Here's how the part is built. I have some questions about the finished solid (model axes, mm). A direction names the side the tool comes from. Round coordinates to 2 decimals unless told otherwise and drop trailing zeros. Loops run counter-clockwise (first coordinate to the right, second up) from the corner with the lowest first, then second, coordinate; pieces in that order, holes last. Notation, with made-up numbers: M 44,-0.5 L 90,-0.5 A22 cw 90,36.5 Z; hole C -33,54.25 d7. An arc over 180 degrees is marked long. One line per question, with ' | ' between items. Start each with the question number.
```python
from build123d import *

# Parameters (mm, degrees)
F0_W     = 76.2
F0_H     = 44.45
F1_DEPTH = 25.4
F2_W     = 25.4
F2_H     = 31.75
F3_DEPTH = 25.4
F5_DEPTH = 25.4
F7_DEPTH = 25.4
F9_DEPTH = 25.4


with BuildPart() as f1:
    # F0 (on Front) → F1 (new body)
    with BuildSketch(Plane.XZ):
        with Locations((38.1, 22.225)):
            Rectangle(F0_W, F0_H)
    extrude(amount=F1_DEPTH)

    # F2 (on face) → F3 (cut)
    with BuildSketch(Plane.XZ.offset(25.4)):
        with Locations((12.7, 28.575)):
            Rectangle(F2_W, F2_H)
        with Locations((63.5, 28.575)):
            Rectangle(F2_W, F2_H)
    extrude(amount=-F3_DEPTH, mode=Mode.SUBTRACT)

    # F4 (on face) → F5 (cut)
    with BuildSketch(Plane.YZ.offset(50.8)):
        with BuildLine():
            Line((-12.7, 28.575), (-12.7, 34.925))
            ThreePointArc((-12.7, 34.925), (-17.1901280605, 33.0651280605), (-19.05, 28.575))
            Line((-19.05, 28.575), (-12.7, 28.575))
        make_face()
        with BuildLine():
            ThreePointArc((-6.35, 28.575), (-8.2098719395, 33.0651280605), (-12.7, 34.925))
            Line((-12.7, 34.925), (-12.7, 28.575))
            Line((-12.7, 28.575), (-6.35, 28.575))
        make_face()
        with BuildLine():
            Line((-6.35, 28.575), (-12.7, 28.575))
            Line((-12.7, 28.575), (-12.7, 22.225))
            ThreePointArc((-12.7, 22.225), (-8.2098719395, 24.0848719395), (-6.35, 28.575))
        make_face()
        with BuildLine():
            Line((-12.7, 22.225), (-12.7, 28.575))
            Line((-12.7, 28.575), (-19.05, 28.575))
            ThreePointArc((-19.05, 28.575), (-17.1901280605, 24.0848719395), (-12.7, 22.225))
        make_face()
        with BuildLine():
            Line((-12.7, 44.3012688375), (-12.7, 44.45))
            Line((-12.7, 44.45), (-25.4, 44.45))
            Line((-25.4, 44.45), (-25.4, 37.8499949622))
            ThreePointArc((-25.4, 37.8499949622), (-19.8223053609, 42.5959948968), (-12.7, 44.3012688375))
        make_face()
        with BuildLine():
            Line((0, 44.45), (-12.7, 44.45))
            Line((-12.7, 44.45), (-12.7, 44.3012688375))
            ThreePointArc((-12.7, 44.3012688375), (-5.5776946391, 42.5959948968), (0, 37.8499949622))
            Line((0, 37.8499949622), (0, 44.45))
        make_face()
    extrude(amount=-F5_DEPTH, mode=Mode.SUBTRACT)

    # F6 (on face) → F7 (cut)
    with BuildSketch(Plane.XY.offset(12.7)):
        with BuildLine():
            Line((6.35, -12.7), (12.7, -12.7))
            Line((12.7, -12.7), (12.7, -6.35))
            ThreePointArc((12.7, -6.35), (8.2098719395, -8.2098719395), (6.35, -12.7))
        make_face()
        with BuildLine():
            Line((12.7, -12.7), (19.05, -12.7))
            ThreePointArc((19.05, -12.7), (17.1901280605, -8.2098719395), (12.7, -6.35))
            Line((12.7, -6.35), (12.7, -12.7))
        make_face()
        with BuildLine():
            Line((12.7, -19.05), (12.7, -12.7))
            Line((12.7, -12.7), (6.35, -12.7))
            ThreePointArc((6.35, -12.7), (8.2098719395, -17.1901280605), (12.7, -19.05))
        make_face()
        with BuildLine():
            ThreePointArc((12.7, -19.05), (17.1901280605, -17.1901280605), (19.05, -12.7))
            Line((19.05, -12.7), (12.7, -12.7))
            Line((12.7, -12.7), (12.7, -19.05))
        make_face()
        with BuildLine():
            ThreePointArc((0, -10.327417444), (4.2938587705, -2.9864667778), (12.2567600012, 0))
            Line((12.2567600012, 0), (0, 0))
            Line((0, 0), (0, -10.327417444))
        make_face()
        with BuildLine():
            Line((0, -25.4), (12.2567600012, -25.4))
            ThreePointArc((12.2567600012, -25.4), (4.2938587705, -22.4135332222), (0, -15.072582556))
            Line((0, -15.072582556), (0, -25.4))
        make_face()
    extrude(amount=-F7_DEPTH, mode=Mode.SUBTRACT)

    # F8 (on face) → F9 (cut)
    with BuildSketch(Plane.XY.offset(12.7)):
        with BuildLine():
            ThreePointArc((63.5, -19.05), (67.9901280605, -17.1901280605), (69.85, -12.7))
            Line((69.85, -12.7), (63.5, -12.7))
            Line((63.5, -12.7), (63.5, -19.05))
        make_face()
        with BuildLine():
            Line((63.5, -12.7), (69.85, -12.7))
            ThreePointArc((69.85, -12.7), (67.9901280605, -8.2098719395), (63.5, -6.35))
            Line((63.5, -6.35), (63.5, -12.7))
        make_face()
        with BuildLine():
            Line((63.5, -19.05), (63.5, -12.7))
            Line((63.5, -12.7), (57.15, -12.7))
            ThreePointArc((57.15, -12.7), (59.0098719395, -17.1901280605), (63.5, -19.05))
        make_face()
        with BuildLine():
            Line((57.15, -12.7), (63.5, -12.7))
            Line((63.5, -12.7), (63.5, -6.35))
            ThreePointArc((63.5, -6.35), (59.0098719395, -8.2098719395), (57.15, -12.7))
        make_face()
        with BuildLine():
            Line((76.2, -25.4), (76.2, -14.4800225697))
            ThreePointArc((76.2, -14.4800225697), (71.9993464021, -22.2483812307), (63.7494866416, -25.4))
            Line((63.7494866416, -25.4), (76.2, -25.4))
        make_face()
        with BuildLine():
            ThreePointArc((63.7494866416, 0), (71.9993464021, -3.1516187693), (76.2, -10.9199774303))
            Line((76.2, -10.9199774303), (76.2, 0))
            Line((76.2, 0), (63.7494866416, 0))
        make_face()
    extrude(amount=-F9_DEPTH, mode=Mode.SUBTRACT)


solid = f1.part
```
1) Imagine slicing it at C-C (y = -18). Write out the boundary of the cut face in (x, z), then the cut area to 3 significant figures.
2) Imagine slicing it at B-B (x = 34). Write out the boundary of the cut face in (y, z) (3 decimals).
3) Imagine slicing it at A-A (z = 7). Write out the boundary of the cut face in (x, y).
4) I'm going to push flat-ended pins straight in: pin 1 Ø2 at (x, y) = (22.5, -16) entering from +Z; pin 2 Ø1 at (y, z) = (-18, 19) entering from -X; pin 3 Ø6 at (x, z) = (67, 7.5) entering from +Y. Where does each tip first touch, or does it pass through?
5) Please list where these lines run through material, in increasing order: L1, parallel to X at y = -20.25, z = 33.5; L2, parallel to Z at x = 53, y = -9.5; L3, parallel to Z at x = 40.5, y = -10.25. Write a range as from..to.
6) For faces 1 (the face through (25.4, -13, 21)), 2 (the face through (50.8, -13, 21)), 3 (the face through (4.4, -22.5, 6.4)), which set-ups out of +Z, -Z, +X, -X, +Y, -Y let a thin tool reach every point of the face, with its end or its side?
7) Imagine slicing it at D-D (x = 14). Write out the boundary of the cut face in (y, z).
Results are:
1) outline: M 0.94,0 L 9.2,0 L 9.2,12.7 L 0.94,12.7 Z; M 16.2,0 L 60,0 L 60,12.7 L 50.8,12.7 L 50.8,25.08 L 25.4,25.08 L 25.4,12.7 L 16.2,12.7 Z; M 25.4,32.07 L 50.8,32.07 L 50.8,43.38 L 25.4,43.38 Z; M 67,0 L 75.17,0 L 75.17,12.7 L 67,12.7 Z | area: 1,370 mm²
2) outline: M -25.4,0 L 0,0 L 0,37.85 A15.726 ccw -25.4,37.85 Z; hole C -12.7,28.575 d12.7
3) outline: M 0,-15.07 A12.7 ccw 12.26,-25.4 L 63.75,-25.4 A12.7 ccw 76.2,-14.48 L 76.2,-10.92 A12.7 ccw 63.75,0 L 12.26,0 A12.7 ccw 0,-10.33 Z; hole C 12.7,-12.7 d12.7; hole C 63.5,-12.7 d12.7
4) pin 1: z = 12.7 | pin 2: x = 25.4 | pin 3: y = 0
5) L1: 25.4..50.8 | L2: 0..12.7 | L3: 0..22.72, 34.43..44.11
6) face 1: +Z, -X, +Y, -Y | face 2: +Z, +X, +Y, -Y | face 3: +Z, -Z, -X, -Y
7) outline: M -25.4,0 L -18.92,0 L -18.92,12.7 L -25.4,12.7 Z; M -6.48,0 L 0,0 L 0,12.7 L -6.48,12.7 Z
